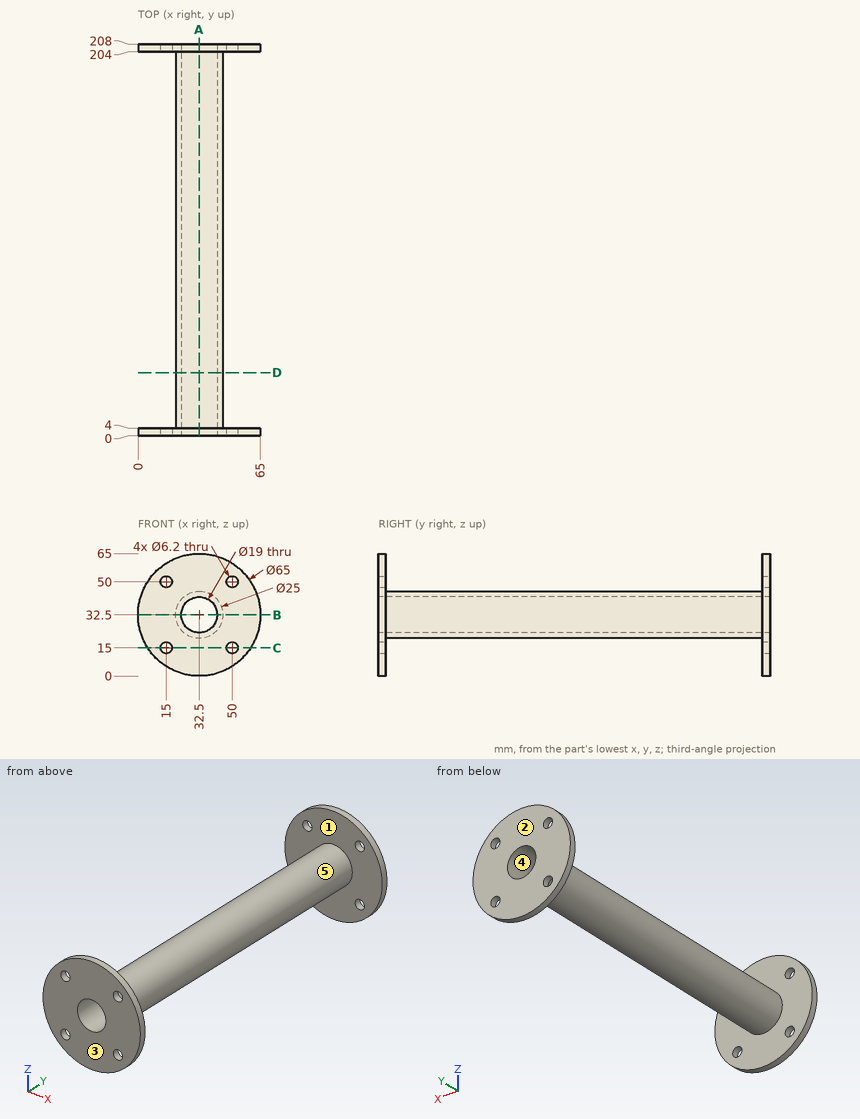
Source: three-view drawing plus pictorial views. Frame: mm from the lowest corner of the part. A direction names the side the tool comes from. Coordinates: 2 decimals unless noted, no trailing zeros. Order: outer loops, then holes, each group sorted by start corner. A loop starts at its lowest first (then second) coordinate and runs counter-clockwise, first axis right, second up. Notation, with made-up numbers: M 20,19 L 36,19 A10 ccw 36,30 Z; hole C 67,-8 d2. An arc over 180 degrees is marked long. Answer in a Markdown table with one row per item.
(1) Section query C-C, the plane z = 15. Output: boundary loops of the cut face in (x, y).
Numbers:
| item | result |
|---|---|
| outline | M 5.11,0 L 11.9,0 L 11.9,4 L 5.11,4 Z; M 5.11,204 L 11.9,204 L 11.9,208 L 5.11,208 Z; M 18.1,0 L 46.9,0 L 46.9,4 L 18.1,4 Z; M 18.1,204 L 46.9,204 L 46.9,208 L 18.1,208 Z; M 53.1,0 L 59.89,0 L 59.89,4 L 53.1,4 Z; M 53.1,204 L 59.89,204 L 59.89,208 L 53.1,208 Z |
(2) Material intervals for line 1 (Y direction, x = 24.5, z = 57.5); line 2 (X direction, y = 1, z = 50); line 3 (X direction, y = 131, z = 35.5), sorted ascending. Write a range as [from, to].
Numbers:
| item | result |
|---|---|
| line 1 | y = [0, 4], [204, 208] |
| line 2 | x = [5.11, 11.9], [18.1, 46.9], [53.1, 59.89] |
| line 3 | x = [20.37, 23.49], [41.51, 44.63] |
(3) Section query D-D, the plane y = 33.5. Output: boundary loops of the cut face in (x, z).
Numbers:
| item | result |
|---|---|
| outline | C 32.5,32.5 d25; hole C 32.5,32.5 d19 |
(4) Section query B-B, the plane z = 32.5. Output: boundary loops of the cut face in (x, y).
Numbers:
| item | result |
|---|---|
| outline | M 0,0 L 23,0 L 23,208 L 0,208 L 0,204 L 20,204 L 20,4 L 0,4 Z; M 42,0 L 65,0 L 65,4 L 45,4 L 45,204 L 65,204 L 65,208 L 42,208 Z |
(5) Section query A-A, the plane x = 32.5. Output: boundary loops of the cut face in (y, z).
Numbers:
| item | result |
|---|---|
| outline | M 0,0 L 4,0 L 4,20 L 204,20 L 204,0 L 208,0 L 208,23 L 0,23 Z; M 0,42 L 208,42 L 208,65 L 204,65 L 204,45 L 4,45 L 4,65 L 0,65 Z |
(6) Draft query along X for the marked faces 3, 4 and 5. Return one class per face: pulls with the +X half, pulls with the -X half, needs draft (parallel to the pull), parting line crosses it, or undercut.
Numbers:
| item | result |
|---|---|
| face 3 | needs draft |
| face 4 | undercut |
| face 5 | parting line crosses it |
(7) Access query for the marked faces 1 and 2. Directions: +Z, -Z, +X, -X, +Y, -Y. A direction counts if a zero-diameter tool reaches every point of the face in a straight line with its end or side. Return the directions, or none.
Numbers:
| item | result |
|---|---|
| face 1 | none |
| face 2 | +Z, -Z, +X, -X, +Y |
(8) Contact query for flat-ended pins moving along their axis: pin 1 Ø8 at (y, z) = (71.5, 22.5) entering from +X; pin 2 Ø2 at (y, z) = (165.5, 27) entering from -X; pin 3 Ø1.5 at (y, z) = (104, 22.5) entering from +X. Output: stop coordinate, or through.
Numbers:
| item | result |
|---|---|
| pin 1 | stops at x = 43.47 |
| pin 2 | stops at x = 20.84 |
| pin 3 | stops at x = 40.91 |
